For this review, take the finished solid that the model builds, in its own axes (mm). A direction names the side the tool comes from. Give positions to 0.01 mm unless a question says otherwise; leave off trailing zeros. Order: outer loops, then holes, each group sorted by start corner. A loop starts at its lowest first (then second) coordinate and runs counter-clockwise, first axis right, second up.
Item 1: For probe 1 along Y at (x, z) = (1071, -1.5); probe 2 along X at (y, z) = (-24.5, -22.5); probe 3 along Y at (x, z) = (729, -4), list the stretches that pass through material, from the lowest coordinate up.
Item 2: Consider section B-B (y = 0). Give the boundary of the cut face in (x, z).
Item 3: Machinability: for faces 1 (the cylindrical face through (31.84, -6.79, -30.59)), 2 (the cylindrical face through (12.522, -0.462, 45.763)), which of the approach directions +Z, -Z, +X, -X, +Y, -Y give a long, thin tool a straight path to every point of the face, cutting with its end or side? Answer none if there is none.
Item 4: The part is to be moulded in two halves that separate along Z. For faces 3 (the cylindrical face through (12.522, 0.462, -45.763)), 4 (the flat face through (13, -31.75, -1)), 5 (the flat face through (101.6, 0, -1)), say which applies: released by +Z, released by -Z, zero draft, split by the parting line, or undercut.
Item 5: Consider section C-C (x = 295.5). Give the boundary of the cut face in (y, z).
Item 6: Consider section A-A (z = 0). Give the boundary of the cut face in (x, y).
Item 7: For P1, Ø19, axis at x = 84, z = -13, coming from the +Y side; P2, Ø1.5, axis at x = 1225.5, y = 7, coming from the +Z side; P3, Ø4, axis at x = 181.5, y = -34.5, coming from the +Z side; P4, Ø11.5, axis at y = -8, z = -36, coming from the +X side, all flat-tipped, find the tip position at first contact; note any pin that passes through.
```python
from build123d import *

# Parameters (mm, degrees)
BOSS_EXTRUDE1_DEPTH = 101.6
SKETCH2_W           = 12.7
SKETCH2_H           = 25.4
SKETCH3_R           = 44.45
SKETCH3_R_2         = 41.91
BOSS_EXTRUDE2_DEPTH = 1524
SKETCH3_2_R         = 44.45
SKETCH3_2_R_2       = 41.91
BOSS_EXTRUDE3_DEPTH = 38.1


with BuildPart() as part:
    # Sketch1 → Boss-Extrude1 (new body)
    with BuildSketch(Plane(origin=(0, 0, 0), x_dir=(0, 0, -1), z_dir=(1, 0, 0))):
        with BuildLine():
            Line((-38.1, 31.75), (38.1, 31.75))
            ThreePointArc((38.1, 31.75), (45.764257606, 0), (38.1, -31.75))
            Line((38.1, -31.75), (-38.1, -31.75))
            ThreePointArc((-38.1, -31.75), (-45.764257606, 0), (-38.1, 31.75))
        make_face()
    extrude(amount=BOSS_EXTRUDE1_DEPTH)

    # Sketch2 → Cut-Revolve1 (revolve, cut)
    with BuildSketch(Plane.XY):
        with Locations((31.75, 44.034385241)):
            Rectangle(SKETCH2_W, SKETCH2_H)
    revolve(axis=Axis((-7.218985368, 0, 0), (1, 0, 0)), mode=Mode.SUBTRACT)

    # Sketch3 → Boss-Extrude2 (add)
    with BuildSketch(Plane(origin=(101.6, 0, 0), x_dir=(0, 0, -1), z_dir=(1, 0, 0))):
        Circle(SKETCH3_R)
        Circle(SKETCH3_R_2, mode=Mode.SUBTRACT)
    extrude(amount=BOSS_EXTRUDE2_DEPTH)

    # Sketch3_2 → Boss-Extrude3 (add)
    with BuildSketch(Plane(origin=(101.6, 0, 0), x_dir=(0, 0, -1), z_dir=(1, 0, 0))):
        Circle(SKETCH3_2_R)
        Circle(SKETCH3_2_R_2, mode=Mode.SUBTRACT)
    extrude(amount=-BOSS_EXTRUDE3_DEPTH)


solid = part.part
```
Resolved:
1. probe 1: y = -44.42 to -41.88, 41.88 to 44.42
1. probe 2: x = 0 to 25.4, 38.1 to 101.6
1. probe 3: y = -44.27 to -41.72, 41.72 to 44.27
2. outline: (0, -45.76) - (25.4, -45.76) - (25.4, -31.33) - (38.1, -31.33) - (38.1, -45.76) - (101.6, -45.76) - (101.6, -44.45) - (1625.6, -44.45) - (1625.6, -41.91) - (101.6, -41.91) - (101.6, 41.91) - (1625.6, 41.91) - (1625.6, 44.45) - (101.6, 44.45) - (101.6, 45.76) - (38.1, 45.76) - (38.1, 31.33) - (25.4, 31.33) - (25.4, 45.76) - (0, 45.76) - close
3. face 1: none
3. face 2: +Z, +X, -X
4. face 3: released by -Z
4. face 4: zero draft
4. face 5: undercut
5. outline: circle Ø88.9 at (0, 0); hole circle Ø83.82 at (0, 0)
6. outline: (0, -31.75) - (25.4, -31.75) - (25.4, -31.33) - (38.1, -31.33) - (38.1, -31.75) - (101.6, -31.75) - (101.6, 31.75) - (38.1, 31.75) - (38.1, 31.33) - (25.4, 31.33) - (25.4, 31.75) - (0, 31.75) - close; (63.5, -44.45) - (1625.6, -44.45) - (1625.6, -41.91) - (63.5, -41.91) - close; (63.5, 41.91) - (1625.6, 41.91) - (1625.6, 44.45) - (63.5, 44.45) - close
7. P1: stops at y = 44.31
7. P2: stops at z = 44.01
7. P3: stops at z = 30.32
7. P4: stops at x = 1625.6
